```python
from build123d import *

# Parameters (mm, degrees)
F1_DEPTH = 6
F2_R     = 3


with BuildPart() as f1:
    # F0 (on Top) → F1 (new body)
    with BuildSketch(Plane.XY):
        Polygon((15, 0), (0, 0), (0, 31.5), (15, 31.5), (15, 36.5), (-5, 36.5), (-5, 0), (-5, -5), (15, -5), align=None)
    extrude(amount=F1_DEPTH)

    # F2
    f2_edges = [f1.edges().sort_by_distance(p)[0] for p in [
        (-5, 36.5, 3),
        (-5, -5, 3),
    ]]
    fillet(f2_edges, radius=F2_R)


solid = f1.part
```
Part model, mm, in its own coordinate system. A direction names the side the tool comes from. Give positions to 0.01 mm unless a question says otherwise; leave off trailing zeros. Loops run counter-clockwise (first coordinate to the right, second up) from the corner with the lowest first, then second, coordinate; pieces in that order, holes last. Notation, with made-up numbers: M -20.5,32.25 L 25.5,32.25 A27 ccw 25.5,68.25 Z; hole C 36.25,33 d4. An arc over 180 degrees is marked long. Return JSON: item names as keys, results as strings.
1) Saw through at A-A, the plane x = 0.5. List the corners of the cut face in (y, z), then the cut area to 3 significant figures.
Calculated:
{"outline": "M -5,0 L 0,0 L 0,6 L -5,6 Z; M 31.5,0 L 36.5,0 L 36.5,6 L 31.5,6 Z", "area": "60.0 mm2"}
2) Saw through at C-C, the plane y = 15. List the corners of the cut face in (x, z), then the cut area to 3 significant figures.
Calculated:
{"outline": "M -5,0 L 0,0 L 0,6 L -5,6 Z", "area": "30.0 mm2"}
3) 3-axis set-ups, long thin cutter, end or side, ignore diameter. For faces 1 (the face through (0, 16, 3)), 2 (the face through (-2, 16, 6)): which of +Z, -Z, +X, -X, +Y, -Y reach the whole face in a straight line?
Calculated:
{"face 1": "+Z, -Z, +X", "face 2": "+Z, +X, -X, +Y, -Y"}
4) Saw through at B-B, the plane z = 2.7. List the corners of the cut face in (x, y), then the cut area to 3 significant figures.
Calculated:
{"outline": "M -5,-2 A3 ccw -2,-5 L 15,-5 L 15,0 L 0,0 L 0,31.5 L 15,31.5 L 15,36.5 L -2,36.5 A3 ccw -5,33.5 Z", "area": "354 mm2"}
5) Flat gauge pin, fed straight in: pin 1 Ø1.5 at (y, z) = (13, 2) entering from +X. Where does the tip first touch, or does it go through?
Calculated:
{"pin 1": "stops at x = 0"}
6) Drill centre lines: line 1 (Y direction, x = 6.25, z = 3.7); line 2 (X direction, y = 6, z = 0.6); line 3 (Y direction, x = -4, z = 0.7). Where is each one in solid material? Low to high.
Calculated:
{"line 1": "y = -5 to 0, 31.5 to 36.5", "line 2": "x = -5 to 0", "line 3": "y = -4.24 to 35.74"}
7) Pull direction Y, two halves, no side cores. Call faces 3 (the face through (15, 34, 3)), 4 (the face through (6, -5, 3)), 5 (the face through (-4.1, 35.64, 3.04)), 6 (the face through (7, 31.5, 3)): released by +Y, released by -Y, zero draft, split by the parting line, or undercut.
Calculated:
{"face 3": "zero draft", "face 4": "released by -Y", "face 5": "released by +Y", "face 6": "undercut"}
